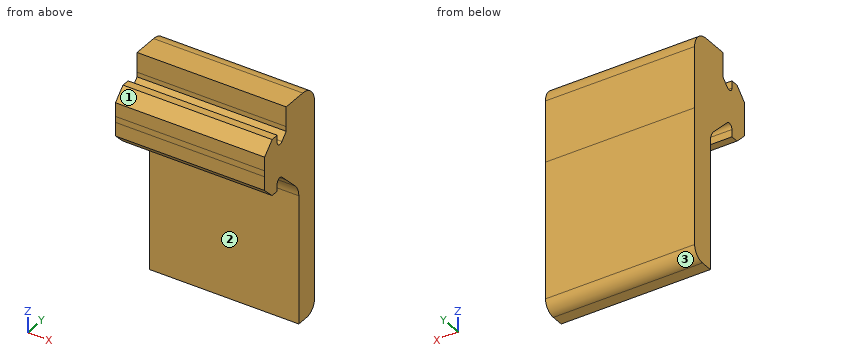
Autodesk Inventor part; units mm, degrees
ref_plane "Work Plane3" through (264.2728, 97.9235, -72.5028) normal (1, 0, 0) x (0, 1, 0)
ref_plane "YZ Plane" through (0, 0, 0) normal (1, 0, 0) x (0, 1, 0)
ref_plane "XZ Plane" through (0, 0, 0) normal (0, 1, 0) x (-1, 0, 0)
ref_plane "Work Plane3" through (264.2728, 97.9235, -72.5028) normal (1, 0, 0) x (0, 1, 0)
sketch "Sketch1" plane through (264.2728, 97.9235, -72.5028) normal (1, 0, 0) x (0, 1, 0)
  line L0 (-1.8, 13.4828) -> (-1.8, 15.2101)
  line L1 (-1.8, 15.2101) -> (-3.8, 15.2101)
  line L2 (-3.8, 15.2101) -> (-6, 13.0101)
  line L3 (-6, 13.0101) -> (-6, 10.5)
  line L4 (-6, 9.5) -> (-6, 6.9899)
  line L5 (-6, 6.9899) -> (-3.8, 4.7899)
  line L6 (-3.8, 4.7899) -> (-1.8, 4.7899)
  line L7 (-1.8, 4.7899) -> (-1.8, 6.5172)
  line L8 (-6, 9.5) -> (-6, 10.5)
  line L9 (-0.0586, 14.7414) -> (-1.4586, 13.3414)
  arc A0 (-1.8, 13.4828) -> (-1.4586, 13.3414) centre (-1.6, 13.4828) ccw
  arc A1 (-1.4586, 6.6586) -> (-1.8, 6.5172) centre (-1.6, 6.5172) ccw
  line L10 (-1.4586, 6.6586) -> (-0.0586, 5.2586)
  line L11 (3.2, 2.7071) -> (-1.105, 7.0121)
  arc A2 (-1.105, 7.0121) -> (-2.3, 6.5172) centre (-1.6, 6.5172) ccw
  line L12 (-2.3, 6.5172) -> (-2.3, 5.2899)
  line L13 (-2.3, 5.2899) -> (-3.5929, 5.2899)
  line L14 (-3.5929, 5.2899) -> (-5.5, 7.1971)
  line L15 (-5.5, 7.1971) -> (-5.5, 9.5)
  line L16 (-5.5, 9.5) -> (-5.5, 10.5)
  line L17 (-5.5, 10.5) -> (-5.5, 12.8029)
  line L18 (-5.5, 12.8029) -> (-3.5929, 14.7101)
  line L19 (-3.5929, 14.7101) -> (-2.3, 14.7101)
  line L20 (-2.3, 14.7101) -> (-2.3, 13.4828)
  arc A3 (-2.3, 13.4828) -> (-1.105, 12.9879) centre (-1.6, 13.4828) ccw
  arc A4 (-0.2, 0) -> (0, 0.2) centre (-0.2, 0.2) ccw
  line L21 (0, 0.2) -> (0, 5.1172)
  arc A5 (0, 5.1172) -> (-0.0586, 5.2586) centre (-0.2, 5.1172) ccw
  line L22 (-1.4586, 6.6586) -> (-0.0586, 5.2586)
  arc A6 (-1.4586, 6.6586) -> (-1.8, 6.5172) centre (-1.6, 6.5172) ccw
  line L23 (-1.8, 4.7899) -> (-1.8, 6.5172)
  line L24 (-3.8, 4.7899) -> (-1.8, 4.7899)
  line L25 (-6, 6.9899) -> (-3.8, 4.7899)
  line L26 (-6, 9.5) -> (-6, 6.9899)
  line L27 (-6.5, 10) -> (-6, 9.5)
  line L28 (-6, 10.5) -> (-6.5, 10)
  line L29 (-6, 13.0101) -> (-6, 10.5)
  line L30 (-3.8, 15.2101) -> (-6, 13.0101)
  line L31 (-1.8, 15.2101) -> (-3.8, 15.2101)
  line L32 (-1.8, 13.4828) -> (-1.8, 15.2101)
  arc A7 (-1.8, 13.4828) -> (-1.4586, 13.3414) centre (-1.6, 13.4828) ccw
  line L33 (-0.0586, 14.7414) -> (-1.4586, 13.3414)
  arc A8 (-0.0586, 14.7414) -> (0, 14.8828) centre (-0.2, 14.8828) ccw
  line L34 (0, 14.8828) -> (0, 19.8)
  arc A9 (0, 19.8) -> (-0.2, 20) centre (-0.2, 19.8) ccw
  line L35 (-0.2, 20) -> (-5.1172, 20)
  arc A10 (-5.1172, 20) -> (-5.2586, 19.9414) centre (-5.1172, 19.8) ccw
  line L36 (-6.6586, 18.5414) -> (-5.2586, 19.9414)
  arc A11 (-6.6586, 18.5414) -> (-6.5172, 18.2) centre (-6.5172, 18.4) ccw
  line L37 (-4.7899, 18.2) -> (-6.5172, 18.2)
  line L38 (-4.7899, 16.2) -> (-4.7899, 18.2)
  line L39 (-6.9899, 14) -> (-4.7899, 16.2)
  line L40 (-9.5, 14) -> (-6.9899, 14)
  line L41 (-10, 13.5) -> (-9.5, 14)
  line L42 (-10.5, 14) -> (-10, 13.5)
  line L43 (-13.0101, 14) -> (-10.5, 14)
  line L44 (-15.2101, 16.2) -> (-13.0101, 14)
  line L45 (-15.2101, 18.2) -> (-15.2101, 16.2)
  line L46 (-13.4828, 18.2) -> (-15.2101, 18.2)
  arc A12 (-13.4828, 18.2) -> (-13.3414, 18.5414) centre (-13.4828, 18.4) ccw
  line L47 (-14.7414, 19.9414) -> (-13.3414, 18.5414)
  arc A13 (-14.7414, 19.9414) -> (-14.8828, 20) centre (-14.8828, 19.8) ccw
  line L48 (-14.8828, 20) -> (-19.8, 20)
  arc A14 (-19.8, 20) -> (-20, 19.8) centre (-19.8, 19.8) ccw
  line L49 (-20, 14.8828) -> (-20, 19.8)
  arc A15 (-20, 14.8828) -> (-19.9414, 14.7414) centre (-19.8, 14.8828) ccw
  line L50 (-18.5414, 13.3414) -> (-19.9414, 14.7414)
  arc A16 (-18.5414, 13.3414) -> (-18.2, 13.4828) centre (-18.4, 13.4828) ccw
  line L51 (-18.2, 15.2101) -> (-18.2, 13.4828)
  line L52 (-16.2, 15.2101) -> (-18.2, 15.2101)
  line L53 (-14, 13.0101) -> (-16.2, 15.2101)
  line L54 (-14, 10.5) -> (-14, 13.0101)
  line L55 (-13.5, 10) -> (-14, 10.5)
  line L56 (-14, 9.5) -> (-13.5, 10)
  line L57 (-14, 6.9899) -> (-14, 9.5)
  line L58 (-16.2, 4.7899) -> (-14, 6.9899)
  line L59 (-18.2, 4.7899) -> (-16.2, 4.7899)
  line L60 (-18.2, 6.5172) -> (-18.2, 4.7899)
  arc A17 (-18.2, 6.5172) -> (-18.5414, 6.6586) centre (-18.4, 6.5172) ccw
  line L61 (-19.9414, 5.2586) -> (-18.5414, 6.6586)
  arc A18 (-19.9414, 5.2586) -> (-20, 5.1172) centre (-19.8, 5.1172) ccw
  line L62 (-20, 0.2) -> (-20, 5.1172)
  arc A19 (-20, 0.2) -> (-19.8, 0) centre (-19.8, 0.2) ccw
  line L63 (-14.8828, 0) -> (-19.8, 0)
  arc A20 (-14.8828, 0) -> (-14.7414, 0.0586) centre (-14.8828, 0.2) ccw
  line L64 (-13.3414, 1.4586) -> (-14.7414, 0.0586)
  arc A21 (-13.3414, 1.4586) -> (-13.4828, 1.8) centre (-13.4828, 1.6) ccw
  line L65 (-15.2101, 1.8) -> (-13.4828, 1.8)
  line L66 (-15.2101, 3.8) -> (-15.2101, 1.8)
  line L67 (-13.0101, 6) -> (-15.2101, 3.8)
  line L68 (-10.5, 6) -> (-13.0101, 6)
  line L69 (-10, 6.5) -> (-10.5, 6)
  line L70 (-9.5, 6) -> (-10, 6.5)
  line L71 (-6.9899, 6) -> (-9.5, 6)
  line L72 (-4.7899, 3.8) -> (-6.9899, 6)
  line L73 (-4.7899, 1.8) -> (-4.7899, 3.8)
  line L74 (-6.5172, 1.8) -> (-4.7899, 1.8)
  arc A22 (-6.5172, 1.8) -> (-6.6586, 1.4586) centre (-6.5172, 1.6) ccw
  line L75 (-5.2586, 0.0586) -> (-6.6586, 1.4586)
  arc A23 (-5.2586, 0.0586) -> (-5.1172, 0) centre (-5.1172, 0.2) ccw
  line L76 (-0.2, 0) -> (-5.1172, 0)
  circle A24 centre (-10, 10) radius 2
  line L77 (0, 5.9071) -> (0, 5.1172)
  line L78 (0.0036, 6) -> (0.0036, 5.9036)
  line L79 (3.2, 2.7071) -> (3.2, -20.1)
  line L80 (0.0036, -20.1) -> (0, -20.1)
  line L81 (0, 1.6971) -> (0, 1.8)
  line L82 (3.2, -20.1) -> (7.2, -20.1)
  line L83 (7.2, -20.1) -> (7.2, 4.9)
  line L84 (7.2, 4.9) -> (7.2, 15.9769)
  line L85 (0, 18.2) -> (7.2, 18.2)
  line L86 (7.2, 18.2) -> (7.2, 15.9769)
  line L87 (0, 18.2) -> (0.0036, 18.1982)
  line L88 (0, 14.8828) -> (0, 14.0929)
  line L89 (0, 14.0929) -> (-1.105, 12.9879)
  dimension "d0" = 0.5
  dimension "d10" = 4
  dimension "d11" = 3.2
extrude "Extrusion1" add sketch "Sketch1" along normal blind 25 contours L34 L85 L86 L84 L83 L82 L79 L11 A2 L12 L13 L14 L15 L16 L17 L18 L19 L20 A3 L89 L88
fillet "Fillet1" radius 3 2 edges at (276.7728, 105.1235, -54.3028) (276.7728, 101.1235, -69.7956)
fillet "Fillet2" radius 2 1 edges at (276.7728, 105.1235, -92.6028)
properties part number "LED Holder"
Source: CAD feature listing. Evaluate the final solid. Frame: model axes, mm. Face numbers are marked on the shaded views. Round coordinates to 2 decimals unless told otherwise and drop trailing zeros. Loops run counter-clockwise (first coordinate to the right, second up) from the corner with the lowest first, then second, coordinate; pieces in that order, holes last. Notation, with made-up numbers: M -1,35 L 16,35 A22 ccw 16,42 Z; hole C -33,50.25 d8. An arc over 180 degrees is marked long. Use a Markdown table: item, result. Add a question column.
1. Cut plane A-A, the plane z = -77.5. Output: boundary loops of the cut face in (x, y).
2. Contact query for flat-ended pins moving along their axis: pin 1 (4 mm diameter, centred on x = 282.5, y = 96.5, fed in from -Z); pin 2 (0.6 mm diameter, centred on x = 277.5, y = 95, fed in from +Z); pin 3 (0.6 mm diameter, centred on x = 280.5, z = -58, fed in from -Y). Output: stop coordinate, or through.
3. Ray query, line 1 along Y through (x, z) = (288, -88); line 2 along Z through (x, y) = (284.75, 96.5); line 3 along Z through (x, y) = (270, 94.5). Return the intervals inside material, ascending. Write a range as [from, to].
4. Pull-direction query (Z, two-part tool) for the marked faces 1, 2 and 3; classes: +Z half, -Z half, draft (parallel to the pull), parting line (faces both ways), or undercut.
5. Cut plane B-B, the plane y = 97.25. Output: boundary loops of the cut face in (x, z), and give its area (3 significant figures).
Solution:
| question | item | result |
|---|---|---|
| 1 | outline | M 264.27,101.12 L 289.27,101.12 L 289.27,105.12 L 264.27,105.12 Z |
| 2 | pin 1 | stops at z = -67.21 |
| 2 | pin 2 | stops at z = -57.79 |
| 2 | pin 3 | stops at y = 93.82 |
| 3 | line 1 | y = [101.12, 105.12] |
| 3 | line 2 | z = [-65.31, -59.7] |
| 3 | line 3 | z = [-67.21, -57.79] |
| 4 | face 1 | +Z half |
| 4 | face 2 | draft |
| 4 | face 3 | -Z half |
| 5 | outline | M 264.27,-65.92 L 289.27,-65.92 L 289.27,-59.08 L 264.27,-59.08 Z |
| 5 | area | 171 mm2 |
